Solid Edge part; units mm, degrees
sketch "Sketch1" plane through (0, 0, 0) normal (0, -1, 0) x (1, 0, 0)
  line L0 (285, 0) -> (295, 60)
  line L1 (295, 60) -> (320, 60)
  line L2 (320, 60) -> (320, 70)
  line L3 (320, 70) -> (286.5287, 70)
  line L4 (286.5287, 70) -> (276.5287, 10)
  line L5 (276.5287, 10) -> (0, 10)
  line L6 (0, 10) -> (0, 0)
  line L7 (0, 0) -> (285, 0)
  dimension "D1" = 320
  dimension "D2" = 295
extrude "Protrusion1" add sketch "Sketch1" against normal blind 20
mirror "Mirror1" about plane through (0, 0, 0) normal (1, 0, 0) of "Protrusion1"
sketch "Sketch2" plane through (287.9289, 10, 70) normal (0, 0, 1) x (1, 0, 0)
  circle A0 centre (-592.3039, 0) radius 5
  circle A1 centre (16.4461, 0) radius 5
extrude "ExtrudedCutout_1" cut sketch "Sketch2" against normal blind 35.7617 and the other way blind 15.9026
The model under review builds one solid part; all positions refer to its coordinate system, in mm. A direction names the side the tool comes from. Round coordinates to 2 decimals unless told otherwise and drop trailing zeros. Write each loop counter-clockwise with the first axis right and the second up, starting at its lowest first coordinate (ties: lowest second). Pieces come first, ordered by that corner, then holes. Notation, with made-up numbers: (0.25, 77) - (37.25, 77) arc R15 cw to (37.25, 103) - close; hole circle Ø7 at (33.5, 70). An arc over 180 degrees is marked (long way). One line per item, written item: value. Start each with the question number.
1. To check wall thickness, follow L1, parallel to Z at x = 51.5, y = 16; L2, parallel to X at y = 3, z = 19.5; L3, parallel to X at y = 15.5, z = 40. State the ranges of each line that lie inside material, in increasing order. Write a range as from..to.
2. Machinability: for faces 1 (the face through (-310, 10, 60)), 2 (the face through (299.8, 7.6, 70)), 3 (the face through (310, 10, 60)), 4 (the face through (-281.46, 9.86, 39.58)), which of the approach directions +Z, -Z, +X, -X, +Y, -Y give a long, thin tool a straight path to every point of the face, cutting with its end or side? Answer none if there is none.
3. Clearance check with flat-ended pins moving along their axes: P1, Ø8, axis at y = 16, z = 51, coming from the -X side; P2, Ø2, axis at y = 3, z = 26.5, coming from the -X side; P3, Ø11.5, axis at x = -304.375, y = 10, coming from the -Z side. State where each tip first meets the part, or that it passes through.
4. Consider section C-C on x = -216.5. Write out the cut boundary in (y, z), and give its area (3 significant figures).
5. The part is to be moulded in two halves that separate along Y. For faces 5 (the face through (1, 0, 9)), 6 (the face through (-299.606, 11.502, 65.07)), 7 (the face through (1, 20, 9)), say which applies: released by +Y, released by -Y, zero draft, split by the parting line, or undercut.
6. Consider section A-A on y = 10. Write out the cut boundary in (x, z) (3 decimals), and give its area (3 significant figures).
7. Consider section B-B on z = 27. Write out the cut boundary in (x, y), and give its area (3 significant figures).
Checks:
1. L1: z = 0..10
1. L2: x = -288.25..-278.11, 278.11..288.25
1. L3: x = -291.67..-281.53, 281.53..291.67
2. face 1: -Z, -X, +Y, -Y
2. face 2: +Z, +X, -X, +Y, -Y
2. face 3: -Z, +X, +Y, -Y
2. face 4: +Z, +Y, -Y
3. P1: stops at x = -294.17
3. P2: stops at x = -289.58
3. P3: stops at z = 60
4. outline: (0, 0) - (20, 0) - (20, 10) - (0, 10) - close
4. area: 200 mm^2
5. face 5: released by -Y
5. face 6: undercut
5. face 7: released by +Y
6. outline: (-320, 60) - (-309.375, 60) - (-309.375, 70) - (-320, 70) - close; (-299.375, 60) - (-295, 60) - (-285, 0) - (285, 0) - (295, 60) - (299.375, 60) - (299.375, 70) - (286.529, 70) - (276.529, 10) - (-276.529, 10) - (-286.529, 70) - (-299.375, 70) - close; (309.375, 60) - (320, 60) - (320, 70) - (309.375, 70) - close
6. area: 7,220 mm^2
7. outline: (-289.5, 0) - (-279.36, 0) - (-279.36, 20) - (-289.5, 20) - close; (279.36, 0) - (289.5, 0) - (289.5, 20) - (279.36, 20) - close
7. area: 406 mm^2
